```python
from build123d import *

# Parameters (mm, degrees)
BOSS_EXTRUDE1_DEPTH = 117.3
SKETCH7_W           = 13.242480008
SKETCH7_H           = 53.740928499
BOSS_EXTRUDE2_DEPTH = 50
SKETCH8_R           = 2.25
CUT_EXTRUDE1_DEPTH  = 13.242480008
SKETCH9_R           = 5.25
SKETCH9_R_2         = 4.930225291
CUT_EXTRUDE2_DEPTH  = 4.5


with BuildPart() as part:
    # Sketch1 → Boss-Extrude1 (new body)
    with BuildSketch(Plane(origin=(0, 0, 0), x_dir=(0, 0, -1), z_dir=(1, 0, 0))):
        with BuildLine():
            Line((0, 0), (81.840140947, 0))
            Line((81.840140947, 0), (81.840140947, 25.960755084))
            Line((81.840140947, 25.960755084), (77.562505861, 25.960755084))
            ThreePointArc((77.562505861, 25.960755084), (65.562505861, 13.960755084), (53.562505861, 25.960755084))
            Line((53.562505861, 25.960755084), (42.320025853, 25.960755084))
            ThreePointArc((42.320025853, 25.960755084), (25.620025853, 9.260755084), (8.920025853, 25.960755084))
            Line((8.920025853, 25.960755084), (0, 25.960755084))
            Line((0, 25.960755084), (0, 0))
        make_face()
    extrude(amount=BOSS_EXTRUDE1_DEPTH)

    # Sketch7 → Boss-Extrude2 (add)
    with BuildSketch(Plane.ZY):
        with Locations((-48.941265857, 26.87046425)):
            Rectangle(SKETCH7_W, SKETCH7_H)
    extrude(amount=BOSS_EXTRUDE2_DEPTH)

    # Sketch8 → Cut-Extrude1 (cut)
    with BuildSketch(Plane(origin=(0, 0, -55.562505861), x_dir=(-1, 0, 0), z_dir=(0, 0, -1))):
        with Locations((12.663905134, 39.560755084)):
            Circle(SKETCH8_R)
        with Locations((12.663905134, 12.360755084)):
            Circle(SKETCH8_R)
    extrude(amount=-CUT_EXTRUDE1_DEPTH, mode=Mode.SUBTRACT)

    # Sketch9 → Cut-Extrude2 (cut)
    with BuildSketch(Plane(origin=(0, 0, -55.562505861), x_dir=(-1, 0, 0), z_dir=(0, 0, -1))):
        with Locations((12.663905134, 39.560755084)):
            Circle(SKETCH9_R)
        with Locations((12.663905134, 12.360755084)):
            Circle(SKETCH9_R_2)
    extrude(amount=-CUT_EXTRUDE2_DEPTH, mode=Mode.SUBTRACT)


solid = part.part
```
Design review of the part built by this model. Coordinates are the model's own, in mm. A direction names the side the tool comes from. Give positions to 0.01 mm unless a question says otherwise; leave off trailing zeros. Order: outer loops, then holes, each group sorted by start corner. A loop starts at its lowest first (then second) coordinate and runs counter-clockwise, first axis right, second up. Notation, with made-up numbers: (-35.75, 6.5) - (-0.75, 6.5) arc R15 ccw to (-0.75, 34.5) - close; hole circle Ø2 at (-3.75, -6). An arc over 180 degrees is marked (long way). Use a Markdown table: item, result. Add a question column.
(1) Add section A-A on x = 82. Give the boundary of the cut face in (y, z).
(2) Mouldability with a two-part tool opening along Z and no side actions: class faces 5 (the face through (-25, 26, -55.563)), 6 (the face through (57.829, 9.265, -25.987)), 7 (the face through (58, 25.961, -48)) as +Z half, -Z half, draft (parallel to the pull), parting line (faces both ways), or undercut.
(3) Wall thickness on probe 1 along Z at (x, y) = (24, 18.5); probe 2 along Z at (x, y) = (59, 20.5); probe 3 along Y at (x, z) = (24, -53): over which ranges is each line inside the solid? List them lowest first. Write a range as [from, to].
(4) Add section B-B on y = 4. Give the boundary of the cut face in (x, z), then the cut area to 3 significant figures.
(5) Clearance check with flat-ended pins moving along their axes: P1, Ø1.3, axis at x = 67.5, z = -80.5, coming from the +Y side; P2, Ø5, axis at x = -11.5, y = 39.5, coming from the -Z side; P3, Ø8, axis at x = -12.66, y = 12.36, coming from the +Z side. State where each tip first meets the part, or that it passes through.
(6) Machinability: for faces 1 (the face through (57.829, 13.964, -65.826)), 2 (the face through (-13, 37, -51.063)), 3 (the face through (0, 10, -69)), 4 (the face through (0, 10, -16)), which of the approach directions +Z, -Z, +X, -X, +Y, -Y give a long, thin tool a straight path to every point of the face, cutting with its end or side? Answer none if there is none.
(7) Add section D-D on z = -6.5. Give the boundary of the cut face in (x, y).
(8) Add section C-C on z = -44.5. Give the boundary of the cut face in (x, y).
Report:
| question | item | result |
|---|---|---|
| 1 | outline | (0, -81.84) - (25.96, -81.84) - (25.96, -77.56) arc R12 cw to (25.96, -53.56) - (25.96, -42.32) arc R16.7 cw to (25.96, -8.92) - (25.96, 0) - (0, 0) - close |
| 2 | face 5 | -Z half |
| 2 | face 6 | undercut |
| 2 | face 7 | draft |
| 3 | probe 1 | z = [-81.84, -74.96], [-56.16, -40.56], [-10.68, 0] |
| 3 | probe 2 | z = [-81.84, -76.25], [-54.88, -41.4], [-9.84, 0] |
| 3 | probe 3 | y = [0, 25.96] |
| 4 | outline | (-50, -55.56) - (0, -55.56) - (0, -81.84) - (117.3, -81.84) - (117.3, 0) - (0, 0) - (0, -42.32) - (-50, -42.32) - close |
| 4 | area | 10,300 mm² |
| 5 | P1 | stops at y = 25.96 |
| 5 | P2 | stops at z = -51.06 |
| 5 | P3 | stops at z = -42.32 |
| 6 | face 1 | +X, +Y |
| 6 | face 2 | -Z |
| 6 | face 3 | -Z, -X, +Y, -Y |
| 6 | face 4 | +Z, -X, +Y, -Y |
| 7 | outline | (0, 0) - (117.3, 0) - (117.3, 25.96) - (0, 25.96) - close |
| 8 | outline | (-50, 0) - (117.3, 0) - (117.3, 25.96) - (0, 25.96) - (0, 53.74) - (-50, 53.74) - close; hole circle Ø4.5 at (-12.66, 12.36); hole circle Ø4.5 at (-12.66, 39.56) |
